Geometry: final body of the model. Coordinates: model frame, mm. A direction names the side the tool comes from. Round coordinates to 2 decimals unless told otherwise and drop trailing zeros. Order: outer loops, then holes, each group sorted by start corner. A loop starts at its lowest first (then second) coordinate and runs counter-clockwise, first axis right, second up. Notation, with made-up numbers: (55.5, 70.25) - (112.5, 70.25) arc R15 ccw to (112.5, 90.25) - close; hole circle Ø2 at (60, 81). An arc over 180 degrees is marked (long way). Put each result on its own line as item: value. Start each with the question number.
(1) Pin query (flat end, axial travel): P1, Ø3, axis at x = -14.5, y = 23, coming from the -Z side; P2, Ø8, axis at x = -11.5, y = 12, coming from the +Z side; P3, Ø2, axis at x = -0.5, y = 1.5, coming from the -Z side; P4, Ø1.5, axis at x = -28.5, z = 22.5, coming from the +Y side. Return the tip coordinate at first contact, or that it passes through.
(2) Material intervals for L1, parallel to Y at x = -15, z = 70.5; L2, parallel to X at y = 15, z = 69.55; L3, parallel to Y at x = -2, z = 21, sorted ascending. Write a range as [from, to].
(3) Section C-C (y = 10). Output: boundary loops of the cut face in (x, z).
(4) Access query for faces 1 (the face through (0, 11, 55)), 2 (the face through (-0.6, 0.6, 80)), 3 (the face through (-15, 28, 69)). Directions: +Z, -Z, +X, -X, +Y, -Y. A direction counts if a zero-diameter tool reaches every point of the face in a straight line with its end or side. Return the directions, or none.
(5) Pull-direction query (Y, two-part tool) for faces 4 (the face through (-15, 15, 71)), 5 (the face through (-29, 15, 34)), 6 (the face through (-15, 0, 45)); classes: released by +Y, released by -Y, zero draft, split by the parting line, or undercut.
(6) Section B-B (x = -9.5). Output: boundary loops of the cut face in (y, z), and give its area (3 significant figures).
(7) Section A-A (z = 67.5). Output: boundary loops of the cut face in (x, y), and give its area (3 significant figures).
from build123d import *

# Parameters (mm, degrees)
SKETCH2_W           = 30
SKETCH2_H           = 30
BOSS_EXTRUDE1_DEPTH = 100
CUT_EXTRUDE1_START  = -30
CUT_EXTRUDE1_DEPTH  = 30
CUT_EXTRUDE2_DEPTH  = 69
CUT_EXTRUDE3_DEPTH  = 80
SKETCH6_R           = 12
CUT_EXTRUDE4_DEPTH  = 2


# Read off the part's stored shape, not the designer's step: Cut-Extrude1
with BuildPart() as part:
    # Sketch2 → Boss-Extrude1 (new body)
    with BuildSketch(Plane.XY):
        with Locations((-15, 15)):
            Rectangle(SKETCH2_W, SKETCH2_H)
    extrude(amount=BOSS_EXTRUDE1_DEPTH)

    # Cut-Extrude1 outline → Cut-Extrude1 (cut)
    with BuildSketch(Plane.XZ.offset(CUT_EXTRUDE1_START)):
        with BuildLine():
            ThreePointArc((-30, 69.824648593), (-16.445900415, 82.511221459), (0, 91.124879576))
            Line((0, 91.124879576), (0, 100))
            Line((0, 100), (-30, 100))
            Line((-30, 100), (-30, 69.824648593))
        make_face()
    extrude(amount=CUT_EXTRUDE1_DEPTH, mode=Mode.SUBTRACT)

    # Sketch4 → Cut-Extrude2 (cut)
    with BuildSketch(Plane(origin=(0, 0, 0), x_dir=(-1, 0, 0), z_dir=(0, 0, -1))):
        with BuildLine():
            Line((3, 15), (0, 15))
            Line((0, 15), (0, 30))
            Line((0, 30), (30, 30))
            Line((30, 30), (30, 15))
            Line((30, 15), (27, 15))
            ThreePointArc((27, 15), (15, 3), (3, 15))
        make_face()
    extrude(amount=-CUT_EXTRUDE2_DEPTH, mode=Mode.SUBTRACT)

    # Sketch5 → Cut-Extrude3 (cut)
    with BuildSketch(Plane(origin=(0, 0, 0), x_dir=(-1, 0, 0), z_dir=(0, 0, -1))):
        Polygon((0, 0), (0, 2), (2, 0), align=None)
    extrude(amount=-CUT_EXTRUDE3_DEPTH, mode=Mode.SUBTRACT)

    # Sketch6 → Cut-Extrude4 (cut)
    with BuildSketch(Plane(origin=(0, 0, 69), x_dir=(-1, 0, 0), z_dir=(0, 0, -1))):
        with Locations((15, 15)):
            Circle(SKETCH6_R)
    extrude(amount=-CUT_EXTRUDE4_DEPTH, mode=Mode.SUBTRACT)


solid = part.part
Checks:
1. P1: stops at z = 71
1. P2: stops at z = 87.89
1. P3: stops at z = 0
1. P4: stops at y = 15
2. L1: y = [0, 3], [27, 30]
2. L2: x = [-30, -27], [-3, 0]
2. L3: y = [0, 15]
3. outline: (-30, 0) - (-25.91, 0) - (-25.91, 71) - (-4.09, 71) - (-4.09, 0) - (0, 0) - (0, 91.12) arc R69 ccw to (-30, 69.82) - close
4. face 1: +Z, -Z, +X, +Y, -Y
4. face 2: -Z, +X, -Y
4. face 3: -Z, +X, -X, +Y
5. face 4: undercut
5. face 5: released by +Y
5. face 6: released by -Y
6. outline: (0, 0) - (4.33, 0) - (4.33, 71) - (25.67, 71) - (25.67, 69) - (30, 69) - (30, 86.85) - (0, 86.85) - close
6. area: 792 mm²
7. outline: (-30, 0) - (-2, 0) - (0, 2) - (0, 15) - (-3, 15) arc R12 cw to (-27, 15) - (-30, 15) - close
7. area: 222 mm²
